Model file for the job. Use its own axes, mm. Face numbers are marked on the shaded views. Round coordinates to 2 decimals unless told otherwise and drop trailing zeros. Order: outer loops, then holes, each group sorted by start corner. A loop starts at its lowest first (then second) coordinate and runs counter-clockwise, first axis right, second up. Notation, with made-up numbers: (59.5, 30) - (68.5, 30) arc R26 ccw to (68.5, 46) - close; hole circle Ø10 at (53.25, -19). An arc over 180 degrees is marked (long way). Use one line per item in the form item = value.
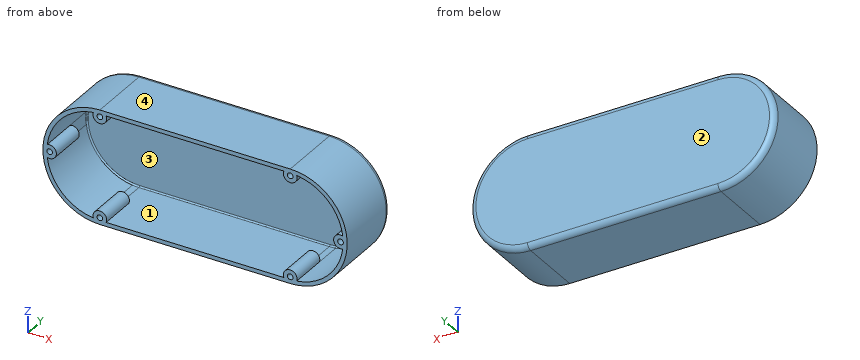
from build123d import *

# Parameters (mm, degrees)
BOSS_EXTRUDE1_DEPTH      = 37
BOSS_EXTRUDE1_DEPTH_BACK = 15
CUT_EXTRUDE1_DEPTH       = 10
CUT_EXTRUDE1_DEPTH_BACK  = 20
SKETCH2_R                = 2.1
FILLET1_R                = 4
SHELL2_START             = -15
SHELL2_DEPTH             = 47.999999899
SHELL2_START_2           = 13
SHELL2_2_DEPTH           = 19.999999899
SHELL2_START_3           = -142
SHELL2_3_DEPTH           = 142
SHELL2_4_ANGLE           = 180
SHELL2_5_ANGLE           = 180


with BuildPart() as part:
    # Sketch1 → Boss-Extrude1 (new, two sides: drawn at the far end of the back side and taken through both)
    with BuildSketch(Plane(origin=(0, 0, 0), x_dir=(1, 0, 0), z_dir=(0, 1, 0)).offset(-BOSS_EXTRUDE1_DEPTH_BACK)):
        with BuildLine():
            Line((0, 42.5), (-142, 42.5))
            ThreePointArc((-142, 42.5), (-184.5, 0), (-142, -42.5))
            Line((-142, -42.5), (0, -42.5))
            ThreePointArc((0, -42.5), (42.5, 0), (0, 42.5))
        make_face()
    extrude(amount=BOSS_EXTRUDE1_DEPTH + BOSS_EXTRUDE1_DEPTH_BACK)

    # Sketch2 → Cut-Extrude1 (cut, two sides: drawn at the far end of the back side and taken through both)
    with BuildSketch(Plane(origin=(0, 0, 0), x_dir=(1, 0, 0), z_dir=(0, 1, 0)).offset(-CUT_EXTRUDE1_DEPTH_BACK)):
        with Locations(Location((-142, 37.5, 0), (0, 0, 270))):
            Circle(SKETCH2_R)
        with Locations(Location((-179.5, 0, 0), (0, 0, 270))):
            Circle(SKETCH2_R)
        with Locations(Location((-142, -37.5, 0), (0, 0, 270))):
            Circle(SKETCH2_R)
        with Locations(Location((0, -37.5, 0), (0, 0, 270))):
            Circle(SKETCH2_R)
        with Locations(Location((37.5, 0, 0), (0, 0, 270))):
            Circle(SKETCH2_R)
        with Locations(Location((0, 37.5, 0), (0, 0, 270))):
            Circle(SKETCH2_R)
    extrude(amount=CUT_EXTRUDE1_DEPTH + CUT_EXTRUDE1_DEPTH_BACK, mode=Mode.SUBTRACT)

    # Fillet1
    fillet1_edges = [part.edges().sort_by_distance(p)[0] for p in [
        (-71, 37, 42.5),
        (42.5, 37, 0),
        (-71, 37, -42.5),
        (-184.5, 37, 0),
    ]]
    fillet(fillet1_edges, radius=FILLET1_R)

    # Shell2: read off the stored shape, not the designer's step
    # Shell2 outline → Shell2 (cut)
    with BuildSketch(Plane(origin=(0, 0, 0), x_dir=(1, 0, 0), z_dir=(0, 1, 0)).offset(SHELL2_START)):
        with BuildLine():
            ThreePointArc((4.806011234, 39.206533333), (-0.157511676, 32.402432926), (-4.691481642, 39.5))
            Line((-4.691481642, 39.5), (-137.308518358, 39.5))
            ThreePointArc((-137.308518358, 39.5), (-141.842488324, 32.402432926), (-146.806011234, 39.206533333))
            ThreePointArc((-146.806011234, 39.206533333), (-169.930717857, 27.930717857), (-181.206533333, 4.806011234))
            ThreePointArc((-181.206533333, 4.806011234), (-174.4, 0), (-181.206533333, -4.806011234))
            ThreePointArc((-181.206533333, -4.806011234), (-169.930717857, -27.930717857), (-146.806011234, -39.206533333))
            ThreePointArc((-146.806011234, -39.206533333), (-141.842488324, -32.402432926), (-137.308518358, -39.5))
            Line((-137.308518358, -39.5), (-4.691481642, -39.5))
            ThreePointArc((-4.691481642, -39.5), (-0.157511676, -32.402432926), (4.806011234, -39.206533333))
            ThreePointArc((4.806011234, -39.206533333), (27.930717857, -27.930717857), (39.206533333, -4.806011234))
            ThreePointArc((39.206533333, -4.806011234), (32.4, 0), (39.206533333, 4.806011234))
            ThreePointArc((39.206533333, 4.806011234), (27.930717857, 27.930717857), (4.806011234, 39.206533333))
        make_face()
    extrude(amount=SHELL2_DEPTH, mode=Mode.SUBTRACT)

    # Shell2 2 outline → Shell2 2 (cut)
    with BuildSketch(Plane(origin=(0, 0, 0), x_dir=(1, 0, 0), z_dir=(0, 1, 0)).offset(SHELL2_START_2)):
        with BuildLine():
            ThreePointArc((4.806011234, 39.206533333), (2.407481395, 39.426565071), (0, 39.5))
            Line((0, 39.5), (-4.691481642, 39.5))
            ThreePointArc((-4.691481642, 39.5), (-0.157511676, 32.402432926), (4.806011234, 39.206533333))
        make_face()
        with BuildLine():
            ThreePointArc((-146.806011234, 39.206533333), (-141.842488324, 32.402432926), (-137.308518358, 39.5))
            Line((-137.308518358, 39.5), (-142, 39.5))
            ThreePointArc((-142, 39.5), (-144.407481395, 39.426565071), (-146.806011234, 39.206533333))
        make_face()
        with BuildLine():
            ThreePointArc((39.206533333, -4.806011234), (39.5, 0), (39.206533333, 4.806011234))
            ThreePointArc((39.206533333, 4.806011234), (32.4, 0), (39.206533333, -4.806011234))
        make_face()
        with BuildLine():
            ThreePointArc((-181.206533333, -4.806011234), (-174.4, 0), (-181.206533333, 4.806011234))
            ThreePointArc((-181.206533333, 4.806011234), (-181.5, 0), (-181.206533333, -4.806011234))
        make_face()
        with BuildLine():
            ThreePointArc((0, -39.5), (2.407481395, -39.426565071), (4.806011234, -39.206533333))
            ThreePointArc((4.806011234, -39.206533333), (-0.157511676, -32.402432926), (-4.691481642, -39.5))
            Line((-4.691481642, -39.5), (0, -39.5))
        make_face()
        with BuildLine():
            ThreePointArc((-137.308518358, -39.5), (-141.842488324, -32.402432926), (-146.806011234, -39.206533333))
            ThreePointArc((-146.806011234, -39.206533333), (-144.407481395, -39.426565071), (-142, -39.5))
            Line((-142, -39.5), (-137.308518358, -39.5))
        make_face()
    extrude(amount=SHELL2_2_DEPTH, mode=Mode.SUBTRACT)

    # Shell2 3 outline → Shell2 3 (cut)
    with BuildSketch(Plane.YZ.offset(SHELL2_START_3)):
        with BuildLine():
            ThreePointArc((33, -39.5), (33.707106781, -39.207106781), (34, -38.5))
            Line((34, -38.5), (34, 38.5))
            ThreePointArc((34, 38.5), (33.707106781, 39.207106781), (33, 39.5))
            Line((33, 39.5), (33, -39.5))
        make_face()
    extrude(amount=SHELL2_3_DEPTH, mode=Mode.SUBTRACT)

    # Shell2 4 outline → Shell2 4 (revolve, cut)
    with BuildSketch(Plane(origin=(-142, 0, 0), x_dir=(0, 0, -1), z_dir=(1, 0, 0))):
        with BuildLine():
            ThreePointArc((39.5, 33), (39.207106781, 33.707106781), (38.5, 34))
            Line((38.5, 34), (0, 34))
            Line((0, 34), (0, 33))
            Line((0, 33), (39.5, 33))
        make_face()
    revolve(axis=Axis((-142, 0, 0), (0, 1, 0)), revolution_arc=SHELL2_4_ANGLE, mode=Mode.SUBTRACT)

    # Shell2 5 outline → Shell2 5 (revolve, cut)
    with BuildSketch(Plane.ZY):
        with BuildLine():
            ThreePointArc((39.5, 33), (39.207106781, 33.707106781), (38.5, 34))
            Line((38.5, 34), (0, 34))
            Line((0, 34), (0, 33))
            Line((0, 33), (39.5, 33))
        make_face()
    revolve(axis=Axis((0, 0, 0), (0, 1, 0)), revolution_arc=SHELL2_5_ANGLE, mode=Mode.SUBTRACT)


solid = part.part
(1) Pin check, flat tips, straight feed: pin 1 (3 mm diameter, centred on x = -94, z = -24.5, fed in from -Y); pin 2 (2 mm diameter, centred on y = 3.5, z = 19.5, fed in from -X); pin 3 (4 mm diameter, centred on y = 10.5, z = -11, fed in from +X). Stop position of each tip, or through.
Report:
pin_1 = 34
pin_2 = -180.26
pin_3 = 41.54
(2) Pull direction Z, two halves, no side cores. Call the marked faces 1, 2, 3 and 4: released by +Z, released by -Z, zero draft, split by the parting line, or undercut.
Report:
face_1 = undercut
face_2 = zero draft
face_3 = undercut
face_4 = released by +Z
(3) Slice it at B-B on x = -43.5. Give the cut face in (y, z), then the cut area to 3 significant figures.
Report:
outline = (-15, -42.5) - (33, -42.5) arc R4 ccw to (37, -38.5) - (37, 38.5) arc R4 ccw to (33, 42.5) - (-15, 42.5) - (-15, 39.5) - (33, 39.5) arc R1 cw to (34, 38.5) - (34, -38.5) arc R1 cw to (33, -39.5) - (-15, -39.5) - close
area = 543 mm2
(4) Probe probe 1 along Z at (x, y) = (-142, 2); probe 2 along Z at (x, y) = (-90.5, -7); probe 3 along X at (y, z) = (3, 0). List the from-to ranges inside material, lowest first. Write a range as [from, to].
Report:
probe_1 = [-42.5, -39.6], [-35.4, -32.4], [32.4, 35.4], [39.6, 42.5]
probe_2 = [-42.5, -39.5], [39.5, 42.5]
probe_3 = [-184.5, -181.6], [-177.4, -174.4], [32.4, 35.4], [39.6, 42.5]
(5) Slice it at A-A on z = 0. Give the cut face in (x, y), then the cut area to 3 significant figures.
Report:
outline = (-184.5, -15) - (-181.6, -15) - (-181.6, 10) - (-177.4, 10) - (-177.4, -15) - (-174.4, -15) - (-174.4, 13) - (-181.5, 13) - (-181.5, 33) arc R1 cw to (-180.5, 34) - (38.5, 34) arc R1 cw to (39.5, 33) - (39.5, 13) - (32.4, 13) - (32.4, -15) - (35.4, -15) - (35.4, 10) - (39.6, 10) - (39.6, -15) - (42.5, -15) - (42.5, 33) arc R4 ccw to (38.5, 37) - (-180.5, 37) arc R4 ccw to (-184.5, 33) - close
area = 1,160 mm2
(6) Slice it at C-C on y = -7. Give the cut face in (x, z).
Report:
outline = (-142, -42.5) - (0, -42.5) arc R42.5 ccw to (0, 42.5) - (-142, 42.5) arc R42.5 ccw to start; hole circle Ø4.2 at (-179.5, 0); hole (-181.21, -4.81) arc R39.5 ccw to (-146.81, -39.21) arc R5.1 cw (long way) to (-137.31, -39.5) - (-4.69, -39.5) arc R5.1 cw (long way) to (4.81, -39.21) arc R39.5 ccw to (39.21, -4.81) arc R5.1 cw (long way) to (39.21, 4.81) arc R39.5 ccw to (4.81, 39.21) arc R5.1 cw (long way) to (-4.69, 39.5) - (-137.31, 39.5) arc R5.1 cw (long way) to (-146.81, 39.21) arc R39.5 ccw to (-181.21, 4.81) arc R5.1 cw (long way) to start; hole circle Ø4.2 at (-142, -37.5); hole circle Ø4.2 at (-142, 37.5); hole circle Ø4.2 at (0, -37.5); hole circle Ø4.2 at (0, 37.5); hole circle Ø4.2 at (37.5, 0)
